The figure shows three views and two pictorial views of one solid part (mm, origin at its lowest corner). Answer the questions. Round coordinates to 2 decimals unless told otherwise and drop trailing zeros. Loops run counter-clockwise (first coordinate to the right, second up) from the corner with the lowest first, then second, coordinate; pieces in that order, holes last. Notation, with made-up numbers: (-35, -13.75) -> (-15, -13.75) arc R30 ccw to (-15, 24.25) -> close; hole circle Ø4 at (-15.5, 75.5). An arc over 180 degrees is marked (long way). Put each result on its own line as item: value.
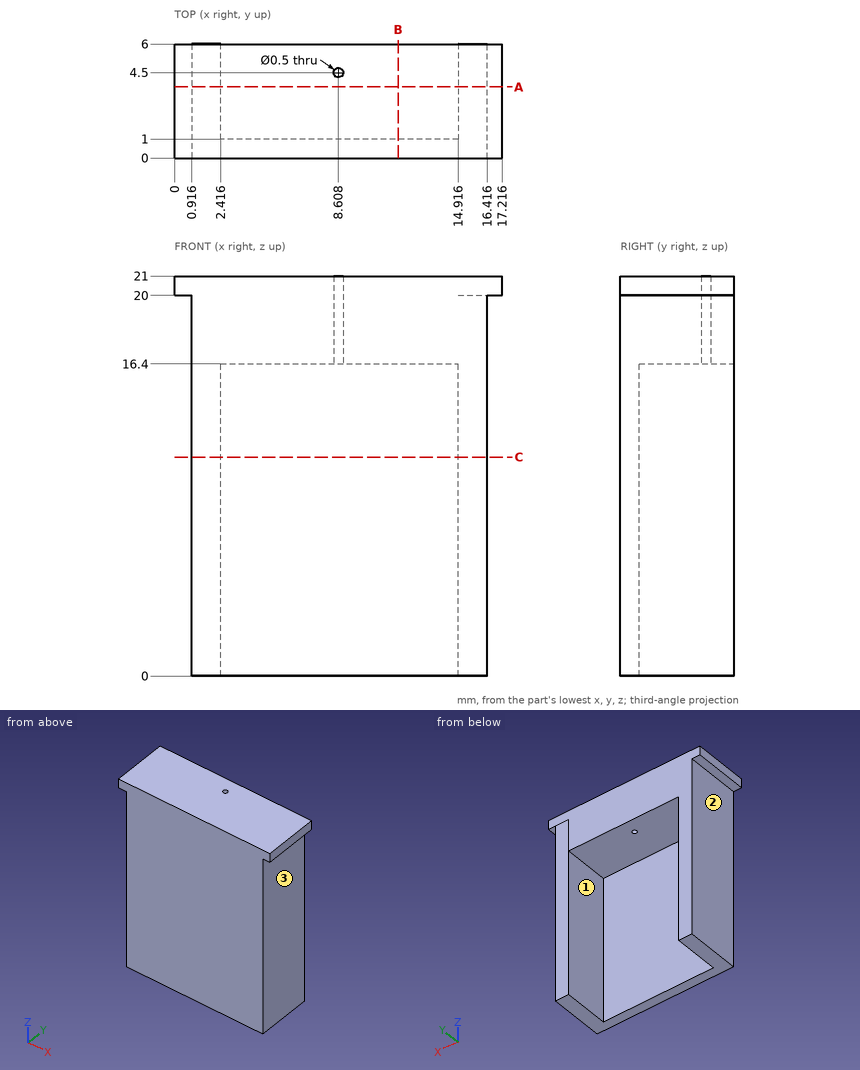
Item 1: Find the intervals of material crossed by line 1 along X through (y, z) = (3.25, 1); line 2 along Z through (x, y) = (8.5, 1.5); line 3 along Y through (x, z) = (10.5, 3.75), in increasing order.
Derived:
line 1: x = 0.92 to 2.42, 14.92 to 16.42
line 2: z = 16.4 to 21
line 3: y = 0 to 1
Item 2: For a pull along X with two mould halves and no side action, classify the marked faces 1, 2 and 3 as pulls with the +X half, pulls with the -X half, needs draft (parallel to the pull), parting line crosses it, or undercut.
Derived:
face 1: undercut
face 2: pulls with the -X half
face 3: pulls with the +X half
Item 3: The part is cut by section C-C (z = 11.5). Determine the outline of the cut face in (x, y).
Derived:
outline: (0.92, 0) -> (16.42, 0) -> (16.42, 6) -> (14.92, 6) -> (14.92, 1) -> (2.42, 1) -> (2.42, 6) -> (0.92, 6) -> close
Item 4: The part is cut by section B-B (x = 11.75). Determine the outline of the cut face in (y, z).
Derived:
outline: (0, 0) -> (1, 0) -> (1, 16.4) -> (6, 16.4) -> (6, 21) -> (0, 21) -> close
Item 5: Flat-ended cylindrical pins translate along their axes: pin 1 Ø1 at (y, z) = (4, 3) entering from -X; pin 2 Ø1 at (x, z) = (4.5, 3.5) entering from +Y; pin 3 Ø2.5 at (x, y) = (7.5, 4) entering from -Z. Find the tip coordinate at first contact, or state that the pin passes through.
Derived:
pin 1: stops at x = 0.92
pin 2: stops at y = 1
pin 3: stops at z = 16.4
Item 6: The part is cut by section A-A (y = 3.75). Determine the outline of the cut face in (x, z), then the cut area to 3 significant figures.
Derived:
outline: (0, 20) -> (0.92, 20) -> (0.92, 0) -> (2.42, 0) -> (2.42, 16.4) -> (14.92, 16.4) -> (14.92, 0) -> (16.42, 0) -> (16.42, 20) -> (17.22, 20) -> (17.22, 21) -> (0, 21) -> close
area: 122 mm^2
